```python
from build123d import *

# Parameters (mm, degrees)
F_0_80_TAPPED_HOLE1_D = 1.19126


with BuildPart() as part:
    # Sketch1 → Revolve1 (revolve)
    with BuildSketch(Plane(origin=(0, 0, 0), x_dir=(0, 0, -1), z_dir=(1, 0, 0)), mode=Mode.PRIVATE) as revolve1_sk:
        Polygon((15.1, 11), (15.1, 7.5436), (13, 7.5436), (13, 5.9436), (0, 5.9436), (0, 7.5436), (11.5, 7.5436), (11.5, 11), align=None)
    revolve(revolve1_sk.sketch.rotate(Axis((0, 0, 0), (0, 0, 1)), 90), axis=Axis((0, 0, 0), (0, 0, 1)))  # turned: the seam where the file's is

    # #0-80 Tapped Hole1 (through all)
    with Locations(Plane(origin=(0, 0, -15.1), x_dir=(-1, 0, 0), z_dir=(0, 0, -1))):
        with Locations((0, 9.2718)):
            f_0_80_tapped_hole1 = Hole(F_0_80_TAPPED_HOLE1_D / 2)

    # Mirror1: #0-80 Tapped Hole1 across plane
    add(f_0_80_tapped_hole1.mirror(Plane.ZX), mode=Mode.SUBTRACT)


solid = part.part
```
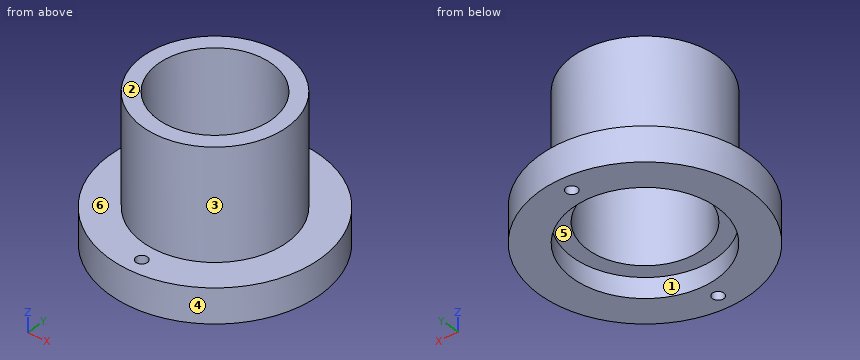
Geometry: final body of the model. Coordinates: model frame, mm. Face numbers are marked on the shaded views. A direction names the side the tool comes from. Coordinates: 2 decimals unless noted, no trailing zeros. Order: outer loops, then holes, each group sorted by start corner. A loop starts at its lowest first (then second) coordinate and runs counter-clockwise, first axis right, second up. Notation, with made-up numbers: M -24.5,25.5 L -19.5,25.5 A18 cw -19.5,45.5 Z; hole C -38,41 d5. An arc over 180 degrees is marked long. Answer in a Markdown table with one row per item. Add a question column.
Q1. Section query B-B on y = 0. Return the cut outline in (x, z), and give its area (3 significant figures).
Q2. Section query A-A on x = 0. Return the cut outline in (y, z), and give its area (3 significant figures).
Q3. Section query C-C on z = -5. Return the cut outline in (x, y).
Q4. Line query: L1, parallel to Y at x = 0, z = -12; L2, parallel to Y at x = 0, z = -13.95; L3, parallel to Z at x = -8.25, y = 0.25. Output: solid intervals per line, ascending.
Q5. Reachability of the marked faces 4, 5 and 6 from +Z, -Z, +X, -X, +Y, -Y: full face, straight path, thin tool, end or side. Return the list, or none.
Q6. Section query D-D on x = 5. Return the cut outline in (y, z), and give its area (3 significant figures).
Q7. Mould query, pull axis Y, two halves, no side actions, for the marked faces 1, 2 and 3. Classes: released by +Y, released by -Y, zero draft, split by the parting line, or undercut.
Q8. Contact query for flat-ended pins moving along their axis: P1, Ø5, axis at x = -7.5, z = -10, coming from the -Y side; P2, Ø1, axis at x = -6.5, z = -7, coming from the +Y side; P3, Ø6, axis at y = 5.5, z = -3.5, coming from the -X side; P4, Ø1.1, axis at x = 0, y = 9.27, coming from the -Z side. Output: stop coordinate, or through.
Completed:
| question | item | result |
|---|---|---|
| 1 | outline | M -11,-15.1 L -7.54,-15.1 L -7.54,-13 L -5.94,-13 L -5.94,0 L -7.54,0 L -7.54,-11.5 L -11,-11.5 Z; M 5.94,-13 L 7.54,-13 L 7.54,-15.1 L 11,-15.1 L 11,-11.5 L 7.54,-11.5 L 7.54,0 L 5.94,0 Z |
| 1 | area | 66.5 mm2 |
| 2 | outline | M -11,-15.1 L -9.87,-15.1 L -9.87,-11.5 L -11,-11.5 Z; M -8.68,-15.1 L -7.54,-15.1 L -7.54,-13 L -5.94,-13 L -5.94,0 L -7.54,0 L -7.54,-11.5 L -8.68,-11.5 Z; M 5.94,-13 L 7.54,-13 L 7.54,-15.1 L 8.68,-15.1 L 8.68,-11.5 L 7.54,-11.5 L 7.54,0 L 5.94,0 Z; M 9.87,-15.1 L 11,-15.1 L 11,-11.5 L 9.87,-11.5 Z |
| 2 | area | 57.9 mm2 |
| 3 | outline | C 0,0 d15.09; hole C 0,0 d11.89 |
| 4 | L1 | y = -11 to -9.87, -8.68 to -5.94, 5.94 to 8.68, 9.87 to 11 |
| 4 | L2 | y = -11 to -9.87, -8.68 to -7.54, 7.54 to 8.68, 9.87 to 11 |
| 4 | L3 | z = -15.1 to -11.5 |
| 5 | face 4 | +Z, -Z |
| 5 | face 5 | -Z |
| 5 | face 6 | +Z |
| 6 | outline | M -9.8,-15.1 L -5.65,-15.1 L -5.65,-13 L -3.21,-13 L -3.21,0 L -5.65,0 L -5.65,-11.5 L -9.8,-11.5 Z; M 3.21,-13 L 5.65,-13 L 5.65,-15.1 L 9.8,-15.1 L 9.8,-11.5 L 5.65,-11.5 L 5.65,0 L 3.21,0 Z |
| 6 | area | 93.2 mm2 |
| 7 | face 1 | undercut |
| 7 | face 2 | zero draft |
| 7 | face 3 | split by the parting line |
| 8 | P1 | stops at y = -9.53 |
| 8 | P2 | stops at y = 4.57 |
| 8 | P3 | stops at x = -7.12 |
| 8 | P4 | passes through |
